Autodesk Inventor part; units mm, degrees
ref_plane "YZ Plane" through (0, 0, 0) normal (1, 0, 0) x (0, 1, 0)
ref_plane "XZ Plane" through (0, 0, 0) normal (0, 1, 0) x (-1, 0, 0)
ref_plane "XY Plane" through (0, 0, 0) normal (0, 0, 1) x (1, 0, 0)
sketch "Boceto1" plane through (0, 0, 0) normal (0, 1, 0) x (-1, 0, 0)
  circle A0 centre (14, 0) radius 1.5
  circle A1 centre (-14, 0) radius 1.5
  line L0 (15, 0) -> (-15, 0) construction
  line L1 (15, 4) -> (-15, 4)
  line L2 (-15, -4) -> (15, -4)
  arc A2 (15, -4) -> (15, 4) centre (15, 0) ccw
  arc A3 (-15, 4) -> (-15, -4) centre (-15, 0) ccw
  line L3 (0, -5.6) -> (0, 5.6)
  circle A4 centre (0, 0) radius 2
  dimension "d2" = 3
  dimension "d3" = 3
  dimension "d4" = 14
  dimension "d5" = 0
  dimension "d6" = 0
  dimension "d7" = 28
  dimension "d8" = 4
  dimension "d9" = 15
  dimension "d12" = 4
extrude "Extrusión2" add sketch "Boceto1" along normal blind 2 contours A2 L2 L3 A4 L1 | L3 A4 L2 A3 L1
properties part number "PINZA_UNION"
Model file for the job. Use its own axes, mm. Coordinates: 2 decimals unless noted, no trailing zeros. Order: outer loops, then holes, each group sorted by start corner. A loop starts at its lowest first (then second) coordinate and runs counter-clockwise, first axis right, second up. Notation, with made-up numbers: M 80.25,51 L 87.25,51 A7 ccw 87.25,58 Z; hole C -24,44 d9. An arc over 180 degrees is marked long. Answer as CSV lines item,"result".
(1) Flat gauge pin, fed straight in: pin 1 (2.5 mm diameter, centred on x = 14, z = 0, fed in from +Y) (1 decimal). Where does the tip first touch, or does it go through?
Geometry says:
pin 1,"passes through"
(2) Band-saw the part on C-C, the plane y = 0.6. List the corners of the cut face in (x, z).
Geometry says:
outline,"M -15,-4 L 15,-4 A4 ccw 15,4 L -15,4 A4 ccw Z; hole C -14,0 d3; hole C 0,0 d4; hole C 14,0 d3"
(3) Pull direction X, two halves, no side cores. Call faces 1 (the cylindrical face through (0, 1, 2)), 2 (the cylindrical face through (-19, 1, 0)), 3 (the flat face through (0, 1, 4)): +X half, -X half, draft (parallel to the pull), parting line (faces both ways), or undercut.
Geometry says:
face 1,"undercut"
face 2,"-X half"
face 3,"draft"
(4) Band-saw the part on D-D, the plane z = -2.5. List the corners of the cut face in (x, y).
Geometry says:
outline,"M -18.12,0 L 18.12,0 L 18.12,2 L -18.12,2 Z"
(5) Band-saw the part on A-A, the plane z = 0. List the corners of the cut face in (x, y).
Geometry says:
outline,"M -19,0 L -15.5,0 L -15.5,2 L -19,2 Z; M -12.5,0 L -2,0 L -2,2 L -12.5,2 Z; M 2,0 L 12.5,0 L 12.5,2 L 2,2 Z; M 15.5,0 L 19,0 L 19,2 L 15.5,2 Z"
(6) Band-saw the part on B-B, the plane x = -14. List the corners of the cut face in (y, z).
Geometry says:
outline,"M 0,-4 L 2,-4 L 2,-1.5 L 0,-1.5 Z; M 0,1.5 L 2,1.5 L 2,4 L 0,4 Z"
(7) Wall check: line 1 along X through (y, z) = (1.25, 0.25); line 2 along Z through (x, y) = (14, 0.9); line 3 along X through (y, z) = (0.5, 0.5). Give the ranges that are in metal, low to high.
Geometry says:
line 1,"x = -18.99 to -15.48, -12.52 to -1.98, 1.98 to 12.52, 15.48 to 18.99"
line 2,"z = -4 to -1.5, 1.5 to 4"
line 3,"x = -18.97 to -15.41, -12.59 to -1.94, 1.94 to 12.59, 15.41 to 18.97"
